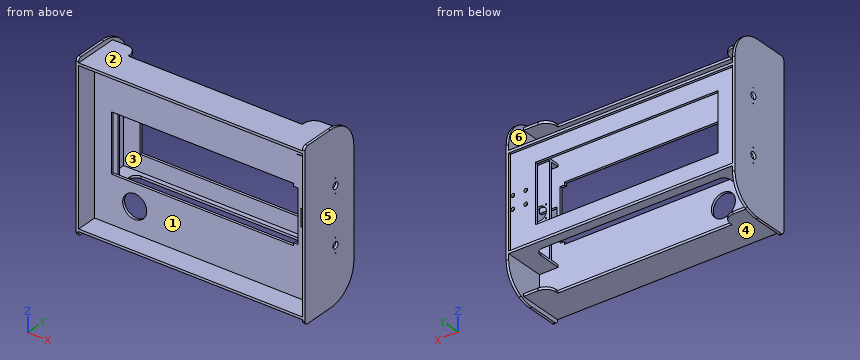
from build123d import *

# Parameters (mm, degrees)
SKETCH_2_W           = 432
SKETCH_2_H           = 220
EXTRUDE_2_DEPTH      = 6
SKETCH_4_W           = 6
SKETCH_4_H           = 28
EXTRUDE_3_DEPTH      = 432
EXTRUDE_4_DEPTH      = 108
SKETCH_6_W           = 540
SKETCH_6_H           = 6
EXTRUDE_5_DEPTH      = 25
EXTRUDE_6_DEPTH      = 6
EXTRUDE_7_DEPTH      = 6
SKETCH_9_W           = 367
SKETCH_9_H           = 6
EXTRUDE_8_DEPTH      = 540
SKETCH_10_R          = 8
CUT_EXTRUDE_1_DEPTH  = 553
SKETCH_11_W          = 6
SKETCH_11_H          = 108
EXTRUDE_9_DEPTH      = 546
SKETCH_12_W          = 70
SKETCH_12_H          = 127
SKETCH_12_W_2        = 195
CUT_EXTRUDE_2_DEPTH  = 6
SKETCH_13_R          = 29
SKETCH_13_W          = 42.3
SKETCH_13_H          = 42.3
CUT_EXTRUDE_3_DEPTH  = 10
SKETCH_14_W          = 220
SKETCH_14_H          = 6
EXTRUDE_10_DEPTH     = 45
SKETCH_15_R          = 16.4
SKETCH_15_R_2        = 1.5
CUT_EXTRUDE_4_DEPTH  = 6
SKETCH_16_R          = 4.5
CUT_EXTRUDE_5_DEPTH  = 6
FILLET_1_R           = 80
FILLET_2_R           = 8
SKETCH_18_W          = 6
SKETCH_18_H          = 75
EXTRUDE_11_DEPTH     = 45
SKETCH_19_W          = 420
SKETCH_19_H          = 30
SKETCH_19_W_2        = 540
CUT_EXTRUDE_8_DEPTH  = 390.5
FILLET_4_R           = 25
FILLET_6_R           = 20
SKETCH_20_W          = 6
SKETCH_20_H          = 75
EXTRUDE_12_DEPTH     = 35
FILLET_7_R           = 15
SKETCH_21_W          = 220
SKETCH_21_H          = 6
EXTRUDE_13_DEPTH     = 35
SKETCH_22_R          = 1
CUT_EXTRUDE_9_DEPTH  = 553
CUT_EXTRUDE_10_DEPTH = 58
SKETCH_24_W          = 440
SKETCH_24_H          = 140
CUT_EXTRUDE_11_DEPTH = 150
SKETCH_25_W          = 309.538461538
SKETCH_25_H          = 30
CUT_EXTRUDE_12_DEPTH = 553
FILLET_8_R           = 70


with BuildPart() as part:
    # Эскиз2 → Бобышка-Вытянуть2 (new body)
    with BuildSketch(Plane(origin=(0, 0, 0), x_dir=(1, 0, 0), z_dir=(0, 1, 0))):
        Rectangle(SKETCH_2_W, SKETCH_2_H)
    extrude(amount=EXTRUDE_2_DEPTH)

    # Эскиз4 → Бобышка-Вытянуть3 (add)
    with BuildSketch(Plane(origin=(216, 0, 0), x_dir=(0, 0, -1), z_dir=(1, 0, 0))):
        with Locations((-113, 3)):
            Rectangle(SKETCH_4_W, SKETCH_4_H)
        with Locations((113, 3)):
            Rectangle(SKETCH_4_W, SKETCH_4_H)
    extrude(amount=-EXTRUDE_3_DEPTH)

    # Эскиз5 → Бобышка-Вытянуть4 (add)
    with BuildSketch(Plane.ZY.offset(216)):
        Polygon((-116, 17), (-110, 17), (-110, 6), (110, 6), (110, 17), (116, 17), (116, -11), (110, -11), (110, 0), (-110, 0), (-110, -11), (-116, -11), align=None)
    extrude(amount=EXTRUDE_4_DEPTH)

    # Эскиз6 → Бобышка-Вытянуть5 (add)
    with BuildSketch(Plane(origin=(0, 17, 0), x_dir=(1, 0, 0), z_dir=(0, 1, 0))):
        with Locations((-54, -113)):
            Rectangle(SKETCH_6_W, SKETCH_6_H)
        with Locations((-54, 113)):
            Rectangle(SKETCH_6_W, SKETCH_6_H)
    extrude(amount=EXTRUDE_5_DEPTH)

    # Эскиз7 → Бобышка-Вытянуть6 (add)
    with BuildSketch(Plane(origin=(216, 0, 0), x_dir=(0, 0, -1), z_dir=(1, 0, 0))):
        Polygon((-200, -143), (-200, -23), (-116, 42), (116, 42), (200, -23), (200, -143), align=None)
    extrude(amount=EXTRUDE_6_DEPTH)

    # Эскиз8 → Бобышка-Вытянуть7 (add)
    with BuildSketch(Plane.ZY.offset(324)):
        Polygon((-116, 42), (-200, -23), (-200, -143), (200, -143), (200, -23), (116, 42), align=None)
    extrude(amount=EXTRUDE_7_DEPTH)

    # Эскиз9 → Бобышка-Вытянуть8 (add)
    with BuildSketch(Plane(origin=(-324, 0, 0), x_dir=(0, 0, -1), z_dir=(1, 0, 0))):
        with Locations((0, -89)):
            Rectangle(SKETCH_9_W, SKETCH_9_H)
    extrude(amount=EXTRUDE_8_DEPTH)

    # Эскиз10 → Вырез-Вытянуть1 (cut, through all)
    with BuildSketch(Plane.ZY.offset(330)):
        with Locations((67, -46.276194705)):
            Circle(SKETCH_10_R)
        with Locations((-67, -46.276194705)):
            Circle(SKETCH_10_R)
    extrude(amount=-CUT_EXTRUDE_1_DEPTH, mode=Mode.SUBTRACT)

    # Эскиз11 → Бобышка-Вытянуть9 (add)
    with BuildSketch(Plane(origin=(222, 0, 0), x_dir=(0, 0, -1), z_dir=(1, 0, 0))):
        with Locations((186.5, -89)):
            Rectangle(SKETCH_11_W, SKETCH_11_H)
        with Locations((-186.5, -89)):
            Rectangle(SKETCH_11_W, SKETCH_11_H)
    extrude(amount=-EXTRUDE_9_DEPTH)

    # Эскиз12 → Вырез-Вытянуть2 (cut)
    with BuildSketch(Plane(origin=(0, -92, 0), x_dir=(-1, 0, 0), z_dir=(0, -1, 0))):
        with Locations((234, 0)):
            Rectangle(SKETCH_12_W, SKETCH_12_H)
        with Locations((51.5, 0)):
            Rectangle(SKETCH_12_W_2, SKETCH_12_H)
        with Locations((-131, 0)):
            Rectangle(SKETCH_12_W, SKETCH_12_H)
    extrude(amount=-CUT_EXTRUDE_2_DEPTH, mode=Mode.SUBTRACT)

    # Эскиз13 → Вырез-Вытянуть3 (cut)
    with BuildSketch(Plane(origin=(0, -86, 0), x_dir=(1, 0, 0), z_dir=(0, 1, 0))):
        with Locations((-227.5, 122.3)):
            Circle(SKETCH_13_R)
        with Locations((194.85, 0)):
            Rectangle(SKETCH_13_W, SKETCH_13_H)
    extrude(amount=-CUT_EXTRUDE_3_DEPTH, mode=Mode.SUBTRACT)

    # Эскиз14 → Бобышка-Вытянуть10 (add)
    with BuildSketch(Plane.ZY.offset(-216)):
        with Locations((0, -61.5)):
            Rectangle(SKETCH_14_W, SKETCH_14_H)
    extrude(amount=EXTRUDE_10_DEPTH)

    # Эскиз15 → Вырез-Вытянуть4 (cut)
    with BuildSketch(Plane(origin=(0, -58.5, 0), x_dir=(1, 0, 0), z_dir=(0, 1, 0))):
        with Locations((194.85, 0)):
            Circle(SKETCH_15_R)
        with Locations((179.35, 15.5)):
            Circle(SKETCH_15_R_2)
        with Locations((210.35, 15.5)):
            Circle(SKETCH_15_R_2)
        with Locations((210.35, -15.5)):
            Circle(SKETCH_15_R_2)
        with Locations((179.35, -15.5)):
            Circle(SKETCH_15_R_2)
    extrude(amount=-CUT_EXTRUDE_4_DEPTH, mode=Mode.SUBTRACT)

    # Эскиз16 → Вырез-Вытянуть5 (cut)
    with BuildSketch(Plane(origin=(0, 6, 0), x_dir=(1, 0, 0), z_dir=(0, 1, 0))):
        with Locations((179.35, 15.5)):
            Circle(SKETCH_16_R)
        with Locations((210.35, 15.5)):
            Circle(SKETCH_16_R)
        with Locations((179.35, -15.5)):
            Circle(SKETCH_16_R)
        with Locations((210.35, -15.5)):
            Circle(SKETCH_16_R)
    extrude(amount=-CUT_EXTRUDE_5_DEPTH, mode=Mode.SUBTRACT)

    # Скругление1
    fillet_1_edges = [part.edges().sort_by_distance(p)[0] for p in [
        (219, -23, -200),
        (219, -23, 200),
        (-327, -23, -200),
        (-327, -23, 200),
    ]]
    fillet(fillet_1_edges, radius=FILLET_1_R)

    # Скругление2
    fillet_2_edges = [part.edges().sort_by_distance(p)[0] for p in [
        (219, -143, 200),
        (219, -143, -200),
        (-327, -143, -200),
        (-327, -143, 200),
    ]]
    fillet(fillet_2_edges, radius=FILLET_2_R)

    # Эскиз18 → Бобышка-Вытянуть11 (add)
    with BuildSketch(Plane.ZY.offset(-216)):
        with Locations((113, -48.5)):
            Rectangle(SKETCH_18_W, SKETCH_18_H)
        with Locations((-113, -48.5)):
            Rectangle(SKETCH_18_W, SKETCH_18_H)
    extrude(amount=EXTRUDE_11_DEPTH)

    # Эскиз19 → Вырез-Вытянуть8 (cut, through all)
    with BuildSketch(Plane.XY.offset(189.5)):
        with Locations((-54, -50)):
            Rectangle(SKETCH_19_W, SKETCH_19_H)
        with Locations((-54, 27)):
            Rectangle(SKETCH_19_W_2, SKETCH_19_H)
    extrude(amount=-CUT_EXTRUDE_8_DEPTH, mode=Mode.SUBTRACT)

    # Скругление4
    fillet_4_edges = [part.edges().sort_by_distance(p)[0] for p in [
        (-264, -35, -186.5),
        (156, -35, -186.5),
        (-264, -35, 186.5),
        (156, -35, 186.5),
    ]]
    fillet(fillet_4_edges, radius=FILLET_4_R)

    # Скругление6
    fillet_6_edges = [part.edges().sort_by_distance(p)[0] for p in [
        (171, -11, 113),
        (171, -11, -113),
    ]]
    fillet(fillet_6_edges, radius=FILLET_6_R)

    # Эскиз20 → Бобышка-Вытянуть12 (add)
    with BuildSketch(Plane(origin=(-324, 0, 0), x_dir=(0, 0, -1), z_dir=(1, 0, 0))):
        with Locations((-113, -48.5)):
            Rectangle(SKETCH_20_W, SKETCH_20_H)
        with Locations((113, -48.5)):
            Rectangle(SKETCH_20_W, SKETCH_20_H)
    extrude(amount=EXTRUDE_12_DEPTH)

    # Скругление7
    fillet_7_edges = [part.edges().sort_by_distance(p)[0] for p in [
        (-289, -11, 113),
        (-289, -11, -113),
    ]]
    fillet(fillet_7_edges, radius=FILLET_7_R)

    # Эскиз21 → Бобышка-Вытянуть13 (add)
    with BuildSketch(Plane(origin=(-324, 0, 0), x_dir=(0, 0, -1), z_dir=(1, 0, 0))):
        with Locations((0, -61.5)):
            Rectangle(SKETCH_21_W, SKETCH_21_H)
    extrude(amount=EXTRUDE_13_DEPTH)

    # Эскиз22 → Вырез-Вытянуть9 (cut, through all)
    with BuildSketch(Plane(origin=(222, 0, 0), x_dir=(0, 0, -1), z_dir=(1, 0, 0))):
        with Locations((84.5, -46.276194705)):
            Circle(SKETCH_22_R)
        with Locations((49.5, -46.276194705)):
            Circle(SKETCH_22_R)
        with Locations((-49.5, -46.276194705)):
            Circle(SKETCH_22_R)
        with Locations((-84.5, -46.276194705)):
            Circle(SKETCH_22_R)
    extrude(amount=-CUT_EXTRUDE_9_DEPTH, mode=Mode.SUBTRACT)

    # Эскиз23 → Вырез-Вытянуть10 (cut, through all)
    with BuildSketch(Plane(origin=(0, -86, 0), x_dir=(1, 0, 0), z_dir=(0, 1, 0))):
        with BuildLine():
            Line((174.514215804, -139.4), (164.514215804, -139.4))
            ThreePointArc((164.514215804, -139.4), (164.014215804, -138.9), (164.514215804, -138.4))
            Line((164.514215804, -138.4), (174.514215804, -138.4))
            ThreePointArc((174.514215804, -138.4), (175.014215804, -138.9), (174.514215804, -139.4))
        make_face()
        with BuildLine():
            Line((174.514215804, -148.9), (164.514215804, -148.9))
            ThreePointArc((164.514215804, -148.9), (164.014215804, -148.4), (164.514215804, -147.9))
            Line((164.514215804, -147.9), (174.514215804, -147.9))
            ThreePointArc((174.514215804, -147.9), (175.014215804, -148.4), (174.514215804, -148.9))
        make_face()
    extrude(amount=-CUT_EXTRUDE_10_DEPTH, mode=Mode.SUBTRACT)

    # Эскиз24 → Вырез-Вытянуть11 (cut, through all)
    with BuildSketch(Plane(origin=(0, 6, 0), x_dir=(1, 0, 0), z_dir=(0, 1, 0))):
        with Locations((-64, 0)):
            Rectangle(SKETCH_24_W, SKETCH_24_H)
    extrude(amount=-CUT_EXTRUDE_11_DEPTH, mode=Mode.SUBTRACT)

    # Эскиз25 → Вырез-Вытянуть12 (cut, through all)
    with BuildSketch(Plane.ZY.offset(330)):
        with Locations((0, 27)):
            Rectangle(SKETCH_25_W, SKETCH_25_H)
    extrude(amount=-CUT_EXTRUDE_12_DEPTH, mode=Mode.SUBTRACT)

    # Скругление8
    fillet_8_edges = [part.edges().sort_by_distance(p)[0] for p in [
        (-327, 12, 154.769230769),
        (-327, 12, -154.769230769),
        (219, 12, -154.769230769),
        (219, 12, 154.769230769),
    ]]
    fillet(fillet_8_edges, radius=FILLET_8_R)


solid = part.part
Can you work these out from the model? Positions are in its coordinate system, mm. Face numbers are marked on the shaded views. A direction names the side the tool comes from. Give positions to 0.01 mm unless a question says otherwise; leave off trailing zeros. Loops run counter-clockwise (first coordinate to the right, second up) from the corner with the lowest first, then second, coordinate; pieces in that order, holes last. Notation, with made-up numbers: (-26.5, -18.75) -> (27.5, -18.75) arc R10 cw to (27.5, -8.75) -> close; hole circle Ø9 at (86, 10). An arc over 180 degrees is marked (long way). Return JSON: item names as keys, results as strings.
Q1. I need wall thicknesses on probe 1 along Z at (x, y) = (210.35, 3.4); probe 2 along Z at (x, y) = (183, -83.5); probe 3 along Y at (x, z) = (-326, 49). Which ranges of each line are inside material? Lowest first, please.
Checks:
{"probe 1": "z = -116 to -20, -11 to 11, 20 to 116", "probe 2": "z = -189.5 to -183.5, -116 to -110, 110 to 116, 183.5 to 189.5", "probe 3": "y = -143 to -47.14, -45.41 to 12"}
Q2. I want a section at D-D, the plane z = 93. List the corners of the cut face in (x, y) for me.
Checks:
{"outline": "(-330, -143) -> (-324, -143) -> (-324, -92) -> (216, -92) -> (216, -143) -> (222, -143) -> (222, 12) -> (216, 12) -> (216, 6) -> (-324, 6) -> (-324, 12) -> (-330, 12) -> close; hole (-324, -86) -> (216, -86) -> (216, -64.5) -> (171, -64.5) -> (171, -58.5) -> (216, -58.5) -> (216, 0) -> (-324, 0) -> (-324, -58.5) -> (-289, -58.5) -> (-289, -64.5) -> (-324, -64.5) -> close"}
Q3. I want a section at A-A, the plane z = -122.3. List the corners of the cut face in (x, y) for me, then the cut area to 3 significant figures.
Checks:
{"outline": "(-330, -143) -> (-324, -143) -> (-324, -92) -> (-256.5, -92) -> (-256.5, -86) -> (-324, -86) -> (-324, 12) -> (-330, 12) -> close; (-198.5, -92) -> (216, -92) -> (216, -143) -> (222, -143) -> (222, 12) -> (216, 12) -> (216, -86) -> (-198.5, -86) -> close", "area": "4,750 mm2"}
Q4. For pin 1 Ø1.8 at (x, y) = (161, -88.5) entering from -Z; pin 2 Ø2.5 at (x, z) = (210.35, 15.5) entering from -Y; pin 3 Ø5 at (x, z) = (-301.5, -187) entering from +Y; pin 4 Ø3 at (x, y) = (-99.5, -122) entering from +Z, each with a flat end and sliding along its axis, tell me the tip position at first contact or that it passes through.
Checks:
{"pin 1": "stops at z = -189.5", "pin 2": "passes through", "pin 3": "stops at y = -35", "pin 4": "stops at z = 189.5"}
Q5. On a 3-axis mill with a long thin cutter (end or side, diameter ignored), from which of +Z, -Z, +X, -X, +Y, -Y can I reach the whole of each face in a straight line? I mean the marked faces 1, 2 and 3. Say none if no direction works.
Checks:
{"face 1": "-Y", "face 2": "+Z, +Y, -Y", "face 3": "none"}
Q6. We'd pull the mould along Z, two halves only. Please class the marked faces 4, 5 and 6: released by +Z, released by -Z, zero draft, split by the parting line, or undercut.
Checks:
{"face 4": "released by -Z", "face 5": "zero draft", "face 6": "undercut"}
Q7. I want a section at B-B, the plane x = 115. Count the separate pieces of the cut face and the enclosed holes in it, then the cut area to 3 significant figures.
Checks:
{"separate pieces": "4", "enclosed holes": "0", "area": "3,050 mm2"}
